Geometry: final body of the model. Coordinates: model frame, mm. A direction names the side the tool comes from. Round coordinates to 2 decimals unless told otherwise and drop trailing zeros. Order: outer loops, then holes, each group sorted by start corner. A loop starts at its lowest first (then second) coordinate and runs counter-clockwise, first axis right, second up. Notation, with made-up numbers: (-1.75, 74) - (32.25, 74) arc R18 cw to (32.25, 101) - close; hole circle Ø3 at (59, -33). An arc over 180 degrees is marked (long way). Put each result on its own line as item: value. Start each with the question number.
(1) Pin query (flat end, axial travel): P1, Ø7.5, axis at x = 3.5, y = 6.5, coming from the -Z side; P2, Ø6, axis at x = 0, z = -29.845, coming from the -Y side; P3, Ø3.5, axis at y = 97.5, z = -18.5, coming from the +X side (3 decimals). Return the tip coordinate at first contact, or that it passes through.
(2) Access query for faces 5 (the face through (0, 74.506, -4)), 6 (the face through (0, 45, -3.175)), 7 (the face through (0, 82, -6.35)). Directions: +Z, -Z, +X, -X, +Y, -Y. A direction counts if a zero-diameter tool reaches every point of the face in a straight line with its end or side. Return the directions, or none.
(3) Pull-direction query (X, two-part tool) for faces 1 (the face through (-6.985, 44, 0)), 2 (the face through (7.3, 85.83, -0.09)), 3 (the face through (12.7, 81, 0)), 4 (the face through (0, 15.24, -4)); classes: released by +X, released by -X, zero draft, split by the parting line, or undercut.
(4) Material intervals for L1, parallel to Y at x = 8.5, z = 2.5; L2, parallel to Y at x = -11.25, z = 3; L3, parallel to Z at x = -8.75, y = 12, sorted ascending. Write a range as [from, to].
(5) Section B-B (z = -29). Output: boundary loops of the cut face in (x, y) (3 decimals), and give its area (3 significant figures).
(6) Section A-A (x = 0). Output: boundary loops of the cut face in (y, z) (3 decimals), and give its area (3 significant figures).
(7) Section C-C (y = 82). Output: boundary loops of the cut face in (x, z), and give its area (3 significant figures).
(8) Section D-D (x = -10.5). Output: boundary loops of the cut face in (y, z), and give its area (3 significant figures).
from build123d import *

# Parameters (mm, degrees)
SKETCH1_W                = 13.97
SKETCH1_H                = 6.35
BOSS_EXTRUDE1_DEPTH      = 95.25
SKETCH3_W                = 25.4
SKETCH3_H                = 13.97
BOSS_EXTRUDE3_DEPTH      = 6.35
BOSS_EXTRUDE5_DEPTH      = 9.525
BOSS_EXTRUDE5_DEPTH_BACK = 9.525
SKETCH5_W                = 12.7
SKETCH5_H                = 15.24
SKETCH6_W                = 13.97
SKETCH6_H                = 38.1
BOSS_EXTRUDE6_DEPTH      = 5.08
SKETCH7_R                = 2.25
CUT_EXTRUDE1_DEPTH       = 5.08
SKETCH8_R                = 0.59563
CUT_EXTRUDE2_DEPTH       = 109.534856843
SKETCH9_R                = 0.889
CUT_EXTRUDE3_DEPTH       = 109.069463309
BOSS_EXTRUDE7_DEPTH      = 6.35
BOSS_EXTRUDE7_DEPTH_BACK = 6.35
SKETCH10_W               = 25.4
SKETCH10_H               = 13.97
SKETCH10_R               = 0.889


with BuildPart() as part:
    # Sketch1 → Boss-Extrude1 (new body)
    with BuildSketch(Plane(origin=(0, 0, 0), x_dir=(1, 0, 0), z_dir=(0, 1, 0))):
        Rectangle(SKETCH1_W, SKETCH1_H)
    extrude(amount=BOSS_EXTRUDE1_DEPTH)

    # Sketch3 → Boss-Extrude3 (add)
    with BuildSketch(Plane.XY.offset(3.175)):
        with Locations((0, 81.491176781)):
            Rectangle(SKETCH3_W, SKETCH3_H)
    extrude(amount=-BOSS_EXTRUDE3_DEPTH)

    # Sketch5 → Boss-Extrude5 (add, two sides: drawn at the far end of the back side and taken through both)
    with BuildSketch(Plane(origin=(0, 0, 0), x_dir=(0, 0, -1), z_dir=(1, 0, 0)).offset(-BOSS_EXTRUDE5_DEPTH_BACK)):
        with Locations((0, 7.62)):
            Rectangle(SKETCH5_W, SKETCH5_H)
    extrude(amount=BOSS_EXTRUDE5_DEPTH + BOSS_EXTRUDE5_DEPTH_BACK)

    # Sketch6 → Boss-Extrude6 (add)
    with BuildSketch(Plane(origin=(0, 95.25, 0), x_dir=(1, 0, 0), z_dir=(0, 1, 0))):
        with Locations((0, 15.875)):
            Rectangle(SKETCH6_W, SKETCH6_H)
    extrude(amount=BOSS_EXTRUDE6_DEPTH)

    # Sketch7 → Cut-Extrude1 (cut)
    with BuildSketch(Plane(origin=(0, 100.33, 0), x_dir=(1, 0, 0), z_dir=(0, 1, 0))):
        with Locations(Location((0, 29.845, 0), (0, 0, 270))):
            Circle(SKETCH7_R)
    extrude(amount=-CUT_EXTRUDE1_DEPTH, mode=Mode.SUBTRACT)

    # Sketch8 → Cut-Extrude2 (cut, through all)
    with BuildSketch(Plane.ZY.offset(9.525)):
        with Locations((-2.286, 12.954)):
            Circle(SKETCH8_R)
        with Locations((2.286, 12.954)):
            Circle(SKETCH8_R)
        with Locations((2.286, 2.286)):
            Circle(SKETCH8_R)
        with Locations((-2.286, 2.286)):
            Circle(SKETCH8_R)
    extrude(amount=-CUT_EXTRUDE2_DEPTH, mode=Mode.SUBTRACT)

    # Sketch9 → Cut-Extrude3 (cut, through all)
    with BuildSketch(Plane.XY.offset(3.175)):
        with Locations((-7.493, 86.698176781)):
            Circle(SKETCH9_R)
        with Locations((7.493, 86.698176781)):
            Circle(SKETCH9_R)
        with Locations((7.493, 76.284176781)):
            Circle(SKETCH9_R)
        with Locations((-7.493, 76.284176781)):
            Circle(SKETCH9_R)
    extrude(amount=-CUT_EXTRUDE3_DEPTH, mode=Mode.SUBTRACT)

    # Sketch10 → Boss-Extrude7 (add, two sides: drawn at the far end of the back side and taken through both)
    with BuildSketch(Plane.XY.offset(-BOSS_EXTRUDE7_DEPTH_BACK)):
        with Locations((0, 81.491176781)):
            Rectangle(SKETCH10_W, SKETCH10_H)
        with Locations((-7.493, 86.698176781)):
            Circle(SKETCH10_R, mode=Mode.SUBTRACT)
        with Locations((-7.493, 76.284176781)):
            Circle(SKETCH10_R, mode=Mode.SUBTRACT)
        with Locations((7.493, 76.284176781)):
            Circle(SKETCH10_R, mode=Mode.SUBTRACT)
        with Locations((7.493, 86.698176781)):
            Circle(SKETCH10_R, mode=Mode.SUBTRACT)
    extrude(amount=BOSS_EXTRUDE7_DEPTH + BOSS_EXTRUDE7_DEPTH_BACK)


solid = part.part
Checks:
1. P1: stops at z = -6.35
1. P2: stops at y = 95.25
1. P3: stops at x = 6.985
2. face 5: none
2. face 6: -Z, +X, -X
2. face 7: -Z, +X, -X, -Y
3. face 1: released by -X
3. face 2: undercut
3. face 3: released by +X
3. face 4: zero draft
4. L1: y = [0, 1.73], [2.84, 12.4], [13.51, 15.24], [74.51, 88.48]
4. L2: y = [74.51, 88.48]
4. L3: z = [-6.35, 6.35]
5. outline: (-6.985, 95.25) - (-2.085, 95.25) - (-2.085, 100.33) - (-6.985, 100.33) - close; (2.085, 95.25) - (6.985, 95.25) - (6.985, 100.33) - (2.085, 100.33) - close
5. area: 49.8 mm²
6. outline: (0, -6.35) - (15.24, -6.35) - (15.24, -3.175) - (74.506, -3.175) - (74.506, -6.35) - (88.476, -6.35) - (88.476, -3.175) - (95.25, -3.175) - (95.25, -27.595) - (100.33, -27.595) - (100.33, 3.175) - (88.476, 3.175) - (88.476, 6.35) - (74.506, 6.35) - (74.506, 3.175) - (15.24, 3.175) - (15.24, 6.35) - (0, 6.35) - close; (95.25, -34.925) - (100.33, -34.925) - (100.33, -32.095) - (95.25, -32.095) - close; hole circle Ø1.191 at (2.286, -2.286); hole circle Ø1.191 at (2.286, 2.286); hole circle Ø1.191 at (12.954, -2.286); hole circle Ø1.191 at (12.954, 2.286)
6. area: 957 mm²
7. outline: (-12.7, -6.35) - (12.7, -6.35) - (12.7, 6.35) - (-12.7, 6.35) - close
7. area: 323 mm²
8. outline: (74.51, -6.35) - (88.48, -6.35) - (88.48, 6.35) - (74.51, 6.35) - close
8. area: 177 mm²
